Can you work these out from the drawing? Everything is in mm from the part's minimum corner. A direction names the side the tool comes from. Give positions to 0.01 mm unless a question says otherwise; leave off trailing zeros. Order: outer loops, then holes, each group sorted by start corner. A loop starts at its lowest first (then second) coordinate and runs counter-clockwise, first axis right, second up. Notation, with made-up numbers: M 70,5.25 L 92,5.25 A30 cw 92,40.25 Z; hole C 18.5,47.5 d11. An arc over 180 degrees is marked long. Use a Markdown table: item, result. Add a question column.
Item 1: For the marked faces 1, 2, 3 and 4, which set-ups out of +Z, -Z, +X, -X, +Y, -Y let a thin tool reach every point of the face, with its end or its side?
Item 2: Suppose I cut it at C-C on y = 15. Write out the boundary of the cut face in (x, z), plus the area to 3 significant figures.
Item 3: If I drill on L1, parallel to X at y = 1.5, z = 7.75; L2, parallel to X at y = 8.5, z = 2.5; L3, parallel to X at y = 5.75, z = 5.25 (1 decimal), over which ranges is the centre line in solid material (lowest first)? Write a range as from..to.
Item 4: I'm going to push flat-ended pins straight in: pin 1 Ø14.5 at (x, y) = (30, 8.49) entering from -Z; pin 2 Ø2.5 at (y, z) = (9.5, 7) entering from -X; pin 3 Ø3 at (x, z) = (36, 3) entering from +Y; pin 4 Ø1.5 at (y, z) = (11, 6.5) entering from +X. Where does each tip first touch, or does it pass through?
Item 5: Suppose I cut it at D-D on z = 7.25. Write out the boundary of the cut face in (x, y).
Item 6: Suppose I cut it at A-A on y = 2. Write out the boundary of the cut face in (x, z).
Item 7: Suppose I cut it at B-B on z = 3.25. Write out the boundary of the cut face in (x, y).
Item 8: If we mould it in two halves opening along X, with no side actions, what happens to the marked faces 5, 6, 7 and 8? For each: released by +X, released by -X, zero draft, split by the parting line, or undercut.
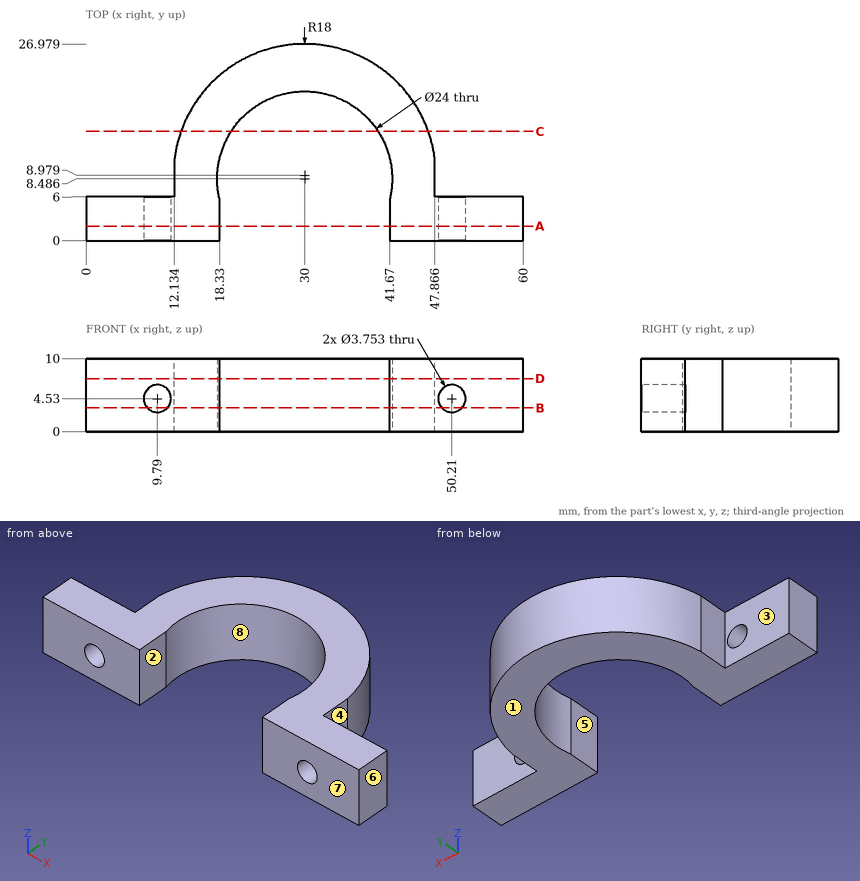
Findings below:
| question | item | result |
|---|---|---|
| 1 | face 1 | -Z, +X, -X, +Y, -Y |
| 1 | face 2 | +Z, -Z, -Y |
| 1 | face 3 | +Z, -Z, -X, +Y |
| 1 | face 4 | +Z, -Z, +X, +Y |
| 2 | outline | M 13.04,0 L 19.92,0 L 19.92,10 L 13.04,10 Z; M 40.08,0 L 46.96,0 L 46.96,10 L 40.08,10 Z |
| 2 | area | 138 mm^2 |
| 3 | L1 | x = 0..18.33, 41.67..60 |
| 3 | L2 | x = 12.13..18, 42..47.87 |
| 3 | L3 | x = 0..8.1, 11.5..18.3, 41.7..48.5, 51.9..60 |
| 4 | pin 1 | passes through |
| 4 | pin 2 | stops at x = 12.13 |
| 4 | pin 3 | stops at y = 26.41 |
| 4 | pin 4 | stops at x = 47.87 |
| 5 | outline | M 0,0 L 18.33,0 L 18.33,5.69 A12 cw long 41.67,5.69 L 41.67,0 L 60,0 L 60,6 L 47.87,6 L 47.87,11.17 A18 ccw 12.13,11.17 L 12.13,6 L 0,6 Z |
| 6 | outline | M 0,0 L 18.33,0 L 18.33,10 L 0,10 Z; M 41.67,0 L 60,0 L 60,10 L 41.67,10 Z; hole C 9.79,4.53 d3.75; hole C 50.21,4.53 d3.75 |
| 7 | outline | M 0,0 L 8.42,0 L 8.42,6 L 0,6 Z; M 11.16,0 L 18.33,0 L 18.33,5.69 A12 cw long 41.67,5.69 L 41.67,0 L 48.84,0 L 48.84,6 L 47.87,6 L 47.87,11.17 A18 ccw 12.13,11.17 L 12.13,6 L 11.16,6 Z; M 51.58,0 L 60,0 L 60,6 L 51.58,6 Z |
| 8 | face 5 | undercut |
| 8 | face 6 | released by +X |
| 8 | face 7 | zero draft |
| 8 | face 8 | undercut |
